```python
from build123d import *

# Parameters (mm, degrees)
SKETCH1_W           = 130
SKETCH1_H           = 97
BOSS_EXTRUDE1_DEPTH = 30
FILLET1_R           = 5
SKETCH2_W           = 70.1
SKETCH2_H           = 55.1
CUT_EXTRUDE3_DEPTH  = 87.471093436


with BuildPart() as part:
    # Sketch1 → Boss-Extrude1 (new body)
    with BuildSketch(Plane(origin=(0, 0, 0), x_dir=(1, 0, 0), z_dir=(0, 1, 0))):
        Rectangle(SKETCH1_W, SKETCH1_H)
    extrude(amount=-BOSS_EXTRUDE1_DEPTH)

    # Fillet1
    fillet1_edges = [part.edges().sort_by_distance(p)[0] for p in [
        (65, -15, 48.5),
        (-65, -15, 48.5),
        (-65, -15, -48.5),
        (65, -15, -48.5),
    ]]
    fillet(fillet1_edges, radius=FILLET1_R)

    # Sketch2 → Cut-Extrude3 (cut, through all)
    with BuildSketch(Plane(origin=(0, -30, 0), x_dir=(1, 0, 0), z_dir=(0, 1, 0))):
        Rectangle(SKETCH2_W, SKETCH2_H)
    extrude(amount=CUT_EXTRUDE3_DEPTH, mode=Mode.SUBTRACT)


solid = part.part
```
For this review, take the finished solid that the model builds, in its own axes (mm). A direction names the side the tool comes from. Round coordinates to 2 decimals unless told otherwise and drop trailing zeros. Order: outer loops, then holes, each group sorted by start corner. A loop starts at its lowest first (then second) coordinate and runs counter-clockwise, first axis right, second up. Notation, with made-up numbers: (53.5, -6) -> (109.5, -6) arc R19 ccw to (109.5, 30) -> close; hole circle Ø7 at (44.5, 84). An arc over 180 degrees is marked (long way). Use a Markdown table: item, result.
Item 1: Take a section at B-B (x = -29). State the section outline as (y, z) points.
Resolved:
| item | result |
|---|---|
| outline | (-30, -48.5) -> (0, -48.5) -> (0, -27.55) -> (-30, -27.55) -> close; (-30, 27.55) -> (0, 27.55) -> (0, 48.5) -> (-30, 48.5) -> close |
Item 2: Take a section at C-C (y = -8.25). State the section outline as (x, z) points, plus the area to 3 significant figures.
Resolved:
| item | result |
|---|---|
| outline | (-65, -43.5) arc R5 ccw to (-60, -48.5) -> (60, -48.5) arc R5 ccw to (65, -43.5) -> (65, 43.5) arc R5 ccw to (60, 48.5) -> (-60, 48.5) arc R5 ccw to (-65, 43.5) -> close; hole (-35.05, -27.55) -> (35.05, -27.55) -> (35.05, 27.55) -> (-35.05, 27.55) -> close |
| area | 8,730 mm² |
Item 3: Machinability: for faces 1 (the flat face through (-35.05, -15, 0)), 2 (the flat face through (-1, 0, -33)), which of the approach directions +Z, -Z, +X, -X, +Y, -Y give a long, thin tool a straight path to every point of the face, cutting with its end or side? Answer none if there is none.
Resolved:
| item | result |
|---|---|
| face 1 | +Y, -Y |
| face 2 | +Z, -Z, +X, -X, +Y |
Item 4: Take a section at A-A (z = 6). State the section outline as (x, y) points, plus the area to 3 significant figures.
Resolved:
| item | result |
|---|---|
| outline | (-65, -30) -> (-35.05, -30) -> (-35.05, 0) -> (-65, 0) -> close; (35.05, -30) -> (65, -30) -> (65, 0) -> (35.05, 0) -> close |
| area | 1,800 mm² |
Item 5: For line 1 along X through (y, z) = (-16.5, 5); line 2 along Z through (x, y) = (-28, -18), list the stretches that pass through material, from the lowest coordinate up. Write a range as [from, to].
Resolved:
| item | result |
|---|---|
| line 1 | x = [-65, -35.05], [35.05, 65] |
| line 2 | z = [-48.5, -27.55], [27.55, 48.5] |
